Input: part model. Units: mm. Frame: model coordinates. Face numbers are marked on the shaded views. A direction names the side the tool comes from. Give positions to 0.01 mm unless a question says otherwise; leave off trailing zeros. Loops run counter-clockwise (first coordinate to the right, second up) from the corner with the lowest first, then second, coordinate; pieces in that order, holes last. Notation, with made-up numbers: (54, -14.75) - (89, -14.75) arc R26 ccw to (89, 17.25) - close; hole circle Ø3 at (-38.5, -23). An arc over 180 degrees is marked (long way). One line per item, written item: value.
from build123d import *

# Parameters (mm, degrees)
SKETCH1_R           = 1.25
BOSS_EXTRUDE1_DEPTH = 11.2
SKETCH2_R           = 0.8
BOSS_EXTRUDE2_DEPTH = 1.5
BOSS_EXTRUDE3_START = -12.7
SKETCH2_2_R         = 0.8
BOSS_EXTRUDE3_DEPTH = 1.5
CHAMFER1_SIZE       = 0.2


with BuildPart() as part:
    # Sketch1 → Boss-Extrude1 (new body)
    with BuildSketch(Plane(origin=(0, 0, 0), x_dir=(1, 0, 0), z_dir=(0, 1, 0))):
        with Locations(Location((0, 0, 0), (0, 0, 270))):
            Circle(SKETCH1_R)
    extrude(amount=BOSS_EXTRUDE1_DEPTH)

    # Sketch2 → Boss-Extrude2 (add)
    with BuildSketch(Plane(origin=(0, 11.2, 0), x_dir=(1, 0, 0), z_dir=(0, 1, 0))):
        with Locations(Location((0, 0, 0), (0, 0, 270))):
            Circle(SKETCH2_R)
    extrude(amount=BOSS_EXTRUDE2_DEPTH)

    # Sketch2<2> → Boss-Extrude3 (add)
    with BuildSketch(Plane(origin=(0, 11.2, 0), x_dir=(1, 0, 0), z_dir=(0, 1, 0)).offset(BOSS_EXTRUDE3_START)):
        with Locations(Location((0, 0, 0), (0, 0, 270))):
            Circle(SKETCH2_2_R)
    extrude(amount=BOSS_EXTRUDE3_DEPTH)

    # Chamfer1
    chamfer1_edges = [part.edges().sort_by_distance(p)[0] for p in [
        (0, -1.5, -0.8),
        (0, 12.7, -0.8),
    ]]
    chamfer(chamfer1_edges, length=CHAMFER1_SIZE)


solid = part.part
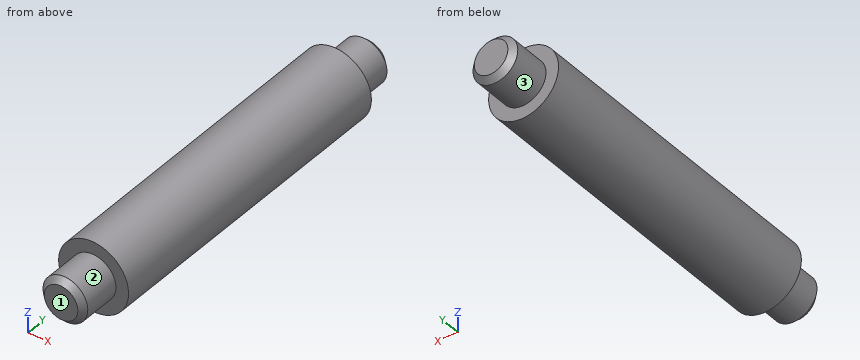
Item 1: Section D-D, the plane z = 1. Output: boundary loops of the cut face in (x, y), and give its area (3 significant figures).
Verdict:
outline: (-0.75, 0) - (0.75, 0) - (0.75, 11.2) - (-0.75, 11.2) - close
area: 16.8 mm^2
Item 2: Section B-B, the plane z = 0. Output: boundary loops of the cut face in (x, y), and give its area (3 significant figures).
Verdict:
outline: (-1.25, 0) - (-0.8, 0) - (-0.8, -1.3) - (-0.6, -1.5) - (0.6, -1.5) - (0.8, -1.3) - (0.8, 0) - (1.25, 0) - (1.25, 11.2) - (0.8, 11.2) - (0.8, 12.5) - (0.6, 12.7) - (-0.6, 12.7) - (-0.8, 12.5) - (-0.8, 11.2) - (-1.25, 11.2) - close
area: 32.7 mm^2
Item 3: Access query for the marked faces 1, 2 and 3. Directions: +Z, -Z, +X, -X, +Y, -Y. A direction counts if a zero-diameter tool reaches every point of the face in a straight line with its end or side. Return the directions, or none.
Verdict:
face 1: +Z, -Z, +X, -X, -Y
face 2: -Y
face 3: +Y
Item 4: Material intervals for L1, parallel to Y at x = 0.2, z = -0.95; L2, parallel to Z at x = -0.8, y = 4; L3, parallel to X at y = 2.5, z = -0.75, sorted ascending.
Verdict:
L1: y = 0 to 11.2
L2: z = -0.96 to 0.96
L3: x = -1 to 1
Item 5: Section C-C, the plane y = 7.5. Output: boundary loops of the cut face in (x, z), and give its area (3 significant figures).
Verdict:
outline: circle Ø2.5 at (0, 0)
area: 4.91 mm^2
Item 6: Section A-A, the plane x = 0. Output: boundary loops of the cut face in (y, z), and give its area (3 significant figures).
Verdict:
outline: (-1.5, -0.6) - (-1.3, -0.8) - (0, -0.8) - (0, -1.25) - (11.2, -1.25) - (11.2, -0.8) - (12.5, -0.8) - (12.7, -0.6) - (12.7, 0.6) - (12.5, 0.8) - (11.2, 0.8) - (11.2, 1.25) - (0, 1.25) - (0, 0.8) - (-1.3, 0.8) - (-1.5, 0.6) - close
area: 32.7 mm^2
